Read the model definition and answer for the solid it produces. Units are mm, in the model's axes. A direction names the side the tool comes from. Give positions to 0.01 mm unless a question says otherwise; leave off trailing zeros. Order: outer loops, then holes, each group sorted by start corner. A loop starts at its lowest first (then second) coordinate and runs counter-clockwise, first axis right, second up.
Item 1: A cutting plane is placed at C-C (z = 2.5). Write down the section's boundary in (x, y).
Item 2: A cutting plane is placed at A-A (y = 0). Write down the section's boundary in (x, z) (1 decimal).
Item 3: A cutting plane is placed at D-D (x = 9.75). Write down the section's boundary in (y, z) (1 decimal), plus the area to 3 significant figures.
Item 4: Given pin 1 Ø5 at (x, y) = (0, 0) entering from +Z (3 decimals); pin 2 Ø3 at (y, z) = (3, -6) entering from +X; pin 3 Ø1.5 at (y, z) = (-3, -1.5) entering from +X, each flat-ended and moving along its own axis, determine where each tip first touches the part or whether it passes through.
Item 5: Find the intervals of material crossed by line 1 along Y through (x, z) = (-0.75, 5); line 2 along X through (y, z) = (0, -3.5) (3 decimals), in increasing order.
Item 6: The mould has two halves that part along X. Classify faces 1 (the face through (-9.803, 9.645, 2.817)), 2 (the face through (9.645, -9.803, 2.898)), 3 (the face through (3, -2, -12.7)), 4 (the face through (-8.057, -8.215, 4.463)): +X half, -X half, draft (parallel to the pull), parting line (faces both ways), or undercut.
Item 7: Which of the six approach directions +Z, -Z, +X, -X, +Y, -Y give full straight-line access (tool end or side, diameter ignored) to faces 5 (the face through (8.145, 6.924, 1.61)), 6 (the face through (7.874, -2.48, -5.478)), 7 (the face through (0, 0, 3.175))?
from build123d import *

# Parameters (mm, degrees)
F0_W     = 25.4
F0_H     = 25.4
F1_DEPTH = 3.175
F2_W     = 25.4
F2_H     = 25.4
F2_W_2   = 22.225
F2_H_2   = 22.225
F3_DEPTH = 2.54
F5_DEPTH = 25.4
F6_R     = 8.255
F6_R_2   = 3.175
F7_DEPTH = 12.7
F8_R     = 10.16
F9_SIZE  = 1.5875


with BuildPart() as f1:
    # F0 (on Top) → F1 (new body)
    with BuildSketch(Plane.XY):
        Rectangle(F0_W, F0_H)
    extrude(amount=F1_DEPTH)

    # F2 (on face) → F3 (join)
    with BuildSketch(Plane.XY.offset(3.175)):
        Rectangle(F2_W, F2_H)
        Rectangle(F2_W_2, F2_H_2, mode=Mode.SUBTRACT)
    extrude(amount=F3_DEPTH)

    # F4 (on face) → F5 (cut)
    with BuildSketch(Plane.XY.offset(3.175)):
        Polygon((7.026218, 4.432465), (9.295024, 9.48628), (4.236917, 7.549808), align=None)
    extrude(amount=-F5_DEPTH, mode=Mode.SUBTRACT)

    # F6 (on face) → F7 (join)
    with BuildSketch(Plane(origin=(0, 0, 0), x_dir=(1, 0, 0), z_dir=(0, 0, -1))):
        Circle(F6_R)
        Circle(F6_R_2, mode=Mode.SUBTRACT)
    extrude(amount=F7_DEPTH)

    # F8
    f8_edges = [f1.edges().sort_by_distance(p)[0] for p in [
        (12.7, -12.7, 2.8575),
        (-12.7, -12.7, 2.8575),
        (-11.1125, -11.1125, 4.445),
        (11.1125, -11.1125, 4.445),
        (-11.1125, 11.1125, 4.445),
        (-12.7, 12.7, 2.8575),
    ]]
    fillet(f8_edges, radius=F8_R)

    # F9
    f9_edges = [f1.edges().sort_by_distance(p)[0] for p in [
        (-8.255, 0, -12.7),
    ]]
    chamfer(f9_edges, length=F9_SIZE)


solid = f1.part
Response values:
1. outline: (-12.7, -2.54) arc R10.16 ccw to (-2.54, -12.7) - (2.54, -12.7) arc R10.16 ccw to (12.7, -2.54) - (12.7, 12.7) - (-2.54, 12.7) arc R10.16 ccw to (-12.7, 2.54) - close; hole (4.24, 7.55) - (7.03, 4.43) - (9.3, 9.49) - close
2. outline: (-12.7, 0) - (-8.3, 0) - (-8.3, -11.1) - (-6.7, -12.7) - (-3.2, -12.7) - (-3.2, 0) - (3.2, 0) - (3.2, -12.7) - (6.7, -12.7) - (8.3, -11.1) - (8.3, 0) - (12.7, 0) - (12.7, 5.7) - (11.1, 5.7) - (11.1, 3.2) - (-11.1, 3.2) - (-11.1, 5.7) - (-12.7, 5.7) - close
3. outline: (-9.7, 0) - (12.7, 0) - (12.7, 5.7) - (11.1, 5.7) - (11.1, 3.2) - (-6, 3.2) - (-6, 5.7) - (-9.7, 5.7) - close
3. area: 84.5 mm2
4. pin 1: stops at z = 3.175
4. pin 2: stops at x = 8.12
4. pin 3: stops at x = 7.94
5. line 1: y = -12.7 to -11.11, 11.11 to 12.7
5. line 2: x = -8.255 to -3.175, 3.175 to 8.255
6. face 1: -X half
6. face 2: +X half
6. face 3: draft
6. face 4: undercut
7. face 5: +Z, -Z
7. face 6: -Z
7. face 7: +Z
